```python
from build123d import *

# Parameters (mm, degrees)
SKETCH1_W                = 125
SKETCH1_H                = 125
BOSS_EXTRUDE1_DEPTH      = 2.5
SKETCH3_W                = 125
SKETCH3_H                = 100
BOSS_EXTRUDE3_DEPTH      = 2.5
SKETCH2_W                = 125
SKETCH2_H                = 100
BOSS_EXTRUDE4_DEPTH      = 2.5
SKETCH5_W                = 125
SKETCH5_H                = 102.5
BOSS_EXTRUDE6_DEPTH      = 2.5
SKETCH11_W               = 8
SKETCH11_H               = 1.5
BOSS_EXTRUDE9_DEPTH      = 3
SKETCH12_W               = 8
SKETCH12_H               = 1.5
BOSS_EXTRUDE10_DEPTH     = 4.5
MIRROR10_COPY_1_SKETCH_W = 8
MIRROR10_COPY_1_SKETCH_H = 1.5
MIRROR10_COPY_1_DEPTH    = 3
MIRROR10_COPY_2_SKETCH_W = 8
MIRROR10_COPY_2_SKETCH_H = 1.5
MIRROR10_COPY_2_DEPTH    = 3
MIRROR11_COPY_1_SKETCH_W = 8
MIRROR11_COPY_1_SKETCH_H = 1.5
MIRROR11_COPY_1_DEPTH    = 4.5
MIRROR11_COPY_2_SKETCH_W = 8
MIRROR11_COPY_2_SKETCH_H = 1.5
MIRROR11_COPY_2_DEPTH    = 4.5
SKETCH13_W               = 3
SKETCH13_H               = 75
CUT_EXTRUDE3_DEPTH       = 4.5
SKETCH15_W               = 3
SKETCH15_H               = 75
CUT_EXTRUDE4_DEPTH       = 4.5
SKETCH17_W               = 3
SKETCH17_H               = 75
CUT_EXTRUDE5_DEPTH       = 4.5
SKETCH18_R               = 1.5
CUT_EXTRUDE6_DEPTH       = 4.5
SKETCH19_R               = 1.5
CUT_EXTRUDE7_DEPTH       = 4.5
SKETCH21_R               = 1.5
CUT_EXTRUDE8_DEPTH       = 4.5
SKETCH20_R               = 1.5
CUT_EXTRUDE9_DEPTH       = 4.5
SKETCH22_R               = 1.5
CUT_EXTRUDE10_DEPTH      = 4.5
SKETCH23_R               = 1.5
CUT_EXTRUDE11_DEPTH      = 4.5
SKETCH24_W               = 125
SKETCH24_H               = 125
BOSS_EXTRUDE11_DEPTH     = 2.5
SKETCH25_W               = 10
SKETCH25_H               = 10
BOSS_EXTRUDE12_DEPTH     = 2.5
SKETCH26_W               = 10
SKETCH26_H               = 10
BOSS_EXTRUDE13_DEPTH     = 2.5
SKETCH27_R               = 1.5
CUT_EXTRUDE12_DEPTH      = 2.5
SKETCH28_R               = 1.5
CUT_EXTRUDE13_DEPTH      = 2.5
SKETCH31_R               = 1.75
CUT_EXTRUDE14_DEPTH      = 10
SKETCH29_R               = 1.75
CUT_EXTRUDE15_DEPTH      = 10
SKETCH32_R               = 1.75
CUT_EXTRUDE16_DEPTH      = 10
FILLET1_R                = 5
FILLET2_R                = 5
SKETCH33_R               = 3.75
CUT_EXTRUDE17_DEPTH      = 10


with BuildPart() as part:
    # Sketch1 → Boss-Extrude1 (new body)
    with BuildSketch(Plane(origin=(0, 0, 0), x_dir=(1, 0, 0), z_dir=(0, 1, 0))):
        Rectangle(SKETCH1_W, SKETCH1_H)
    extrude(amount=BOSS_EXTRUDE1_DEPTH)

    # Sketch3 → Boss-Extrude3 (add)
    with BuildSketch(Plane(origin=(0, 0, -62.5), x_dir=(-1, 0, 0), z_dir=(0, 0, -1))):
        with Locations((0, 52.5)):
            Rectangle(SKETCH3_W, SKETCH3_H)
    extrude(amount=-BOSS_EXTRUDE3_DEPTH)

    # Sketch2 → Boss-Extrude4 (add)
    with BuildSketch(Plane.XY.offset(62.5)):
        with Locations((0, 52.5)):
            Rectangle(SKETCH2_W, SKETCH2_H)
    extrude(amount=-BOSS_EXTRUDE4_DEPTH)

    # Sketch5 → Boss-Extrude6 (add)
    with BuildSketch(Plane(origin=(62.5, 0, 0), x_dir=(0, 0, -1), z_dir=(1, 0, 0))):
        with Locations((0, 51.25)):
            Rectangle(SKETCH5_W, SKETCH5_H)
    extrude(amount=-BOSS_EXTRUDE6_DEPTH)

    # Sketch11 → Boss-Extrude9 (add)
    with BuildSketch(Plane(origin=(0, 2.5, 0), x_dir=(1, 0, 0), z_dir=(0, 1, 0))):
        with Locations((54, 50.75)):
            Rectangle(SKETCH11_W, SKETCH11_H)
    boss_extrude9 = extrude(amount=BOSS_EXTRUDE9_DEPTH)

    # Mirror6: Boss-Extrude9 across plane
    add(boss_extrude9.mirror(Plane.XY))

    # Sketch12 → Boss-Extrude10 (add)
    with BuildSketch(Plane.XY.offset(-50)):
        with Locations((54, 4.75)):
            Rectangle(SKETCH12_W, SKETCH12_H)
    boss_extrude10 = extrude(amount=BOSS_EXTRUDE10_DEPTH)

    # Mirror7: Boss-Extrude10 across plane
    add(boss_extrude10.mirror(Plane.XY))

    # Mirror8: Boss-Extrude9 across plane
    add(boss_extrude9.mirror(Plane(origin=(0, 0, 0), x_dir=(0, 0, 1), z_dir=(1, 0, 0))))

    # Mirror9: Boss-Extrude10 across plane
    add(boss_extrude10.mirror(Plane(origin=(0, 0, 0), x_dir=(0, 0, 1), z_dir=(1, 0, 0))))

    # Mirror10 copy 1 sketch → Mirror10 copy 1 (add)
    with BuildSketch(Plane(origin=(0, 2.5, 0), x_dir=(-1, 0, 0), z_dir=(0, 1, 0))):
        with Locations((54, 50.75)):
            Rectangle(MIRROR10_COPY_1_SKETCH_W, MIRROR10_COPY_1_SKETCH_H)
    extrude(amount=MIRROR10_COPY_1_DEPTH)

    # Mirror10 copy 2 sketch → Mirror10 copy 2 (add)
    with BuildSketch(Plane(origin=(0, 2.5, 0), x_dir=(1, 0, 0), z_dir=(0, 1, 0))):
        with Locations((54, -50.75)):
            Rectangle(MIRROR10_COPY_2_SKETCH_W, MIRROR10_COPY_2_SKETCH_H)
    extrude(amount=MIRROR10_COPY_2_DEPTH)

    # Mirror11 copy 1 sketch → Mirror11 copy 1 (add)
    with BuildSketch(Plane(origin=(0, 0, 50), x_dir=(-1, 0, 0), z_dir=(0, 0, -1))):
        with Locations((54, 4.75)):
            Rectangle(MIRROR11_COPY_1_SKETCH_W, MIRROR11_COPY_1_SKETCH_H)
    extrude(amount=MIRROR11_COPY_1_DEPTH)

    # Mirror11 copy 2 sketch → Mirror11 copy 2 (add)
    with BuildSketch(Plane(origin=(0, 0, 50), x_dir=(1, 0, 0), z_dir=(0, 0, -1))):
        with Locations((54, -4.75)):
            Rectangle(MIRROR11_COPY_2_SKETCH_W, MIRROR11_COPY_2_SKETCH_H)
    extrude(amount=MIRROR11_COPY_2_DEPTH)

    # Sketch13 → Cut-Extrude3 (cut)
    with BuildSketch(Plane(origin=(62.5, 0, -52.868964846), x_dir=(0, 0, -1), z_dir=(1, 0, 0))):
        with Locations((-61.5, 52.5)):
            Rectangle(SKETCH13_W, SKETCH13_H)
    cut_extrude3 = extrude(amount=-CUT_EXTRUDE3_DEPTH, mode=Mode.SUBTRACT)

    # Sketch15 → Cut-Extrude4 (cut)
    with BuildSketch(Plane(origin=(62.5, 0, 0), x_dir=(0, 0, -1), z_dir=(1, 0, 0))):
        with Locations((-43.5, 52.5)):
            Rectangle(SKETCH15_W, SKETCH15_H)
    cut_extrude4 = extrude(amount=-CUT_EXTRUDE4_DEPTH, mode=Mode.SUBTRACT)

    # Sketch17 → Cut-Extrude5 (cut)
    with BuildSketch(Plane(origin=(62.5, 0, 0), x_dir=(0, 0, -1), z_dir=(1, 0, 0))):
        with Locations((-26, 52.5)):
            Rectangle(SKETCH17_W, SKETCH17_H)
    cut_extrude5 = extrude(amount=-CUT_EXTRUDE5_DEPTH, mode=Mode.SUBTRACT)

    # Mirror12: Cut-Extrude5 across plane
    add(cut_extrude5.mirror(Plane.XY), mode=Mode.SUBTRACT)

    # Mirror13: Cut-Extrude4 across plane
    add(cut_extrude4.mirror(Plane.XY), mode=Mode.SUBTRACT)

    # Mirror14: Cut-Extrude3 across plane
    add(cut_extrude3.mirror(Plane.XY), mode=Mode.SUBTRACT)

    # Sketch18 → Cut-Extrude6 (cut)
    with BuildSketch(Plane(origin=(62.5, 0, 0), x_dir=(0, 0, -1), z_dir=(1, 0, 0))):
        with Locations((-8.631035154, 90)):
            Circle(SKETCH18_R)
    cut_extrude6 = extrude(amount=-CUT_EXTRUDE6_DEPTH, mode=Mode.SUBTRACT)

    # Sketch19 → Cut-Extrude7 (cut)
    with BuildSketch(Plane(origin=(62.5, 0, 0), x_dir=(0, 0, -1), z_dir=(1, 0, 0))):
        with Locations((-8.631035154, 15)):
            Circle(SKETCH19_R)
    cut_extrude7 = extrude(amount=-CUT_EXTRUDE7_DEPTH, mode=Mode.SUBTRACT)

    # Sketch21 → Cut-Extrude8 (cut)
    with BuildSketch(Plane(origin=(62.5, 0, 0), x_dir=(0, 0, -1), z_dir=(1, 0, 0))):
        with Locations((-26, 15)):
            Circle(SKETCH21_R)
    cut_extrude8 = extrude(amount=-CUT_EXTRUDE8_DEPTH, mode=Mode.SUBTRACT)

    # Sketch20 → Cut-Extrude9 (cut)
    with BuildSketch(Plane(origin=(62.5, 0, 0), x_dir=(0, 0, -1), z_dir=(1, 0, 0))):
        with Locations((-43.5, 15)):
            Circle(SKETCH20_R)
    cut_extrude9 = extrude(amount=-CUT_EXTRUDE9_DEPTH, mode=Mode.SUBTRACT)

    # Mirror15: Cut-Extrude7 across plane
    add(cut_extrude7.mirror(Plane.XY), mode=Mode.SUBTRACT)

    # Mirror16: Cut-Extrude9 across plane
    add(cut_extrude9.mirror(Plane.XY), mode=Mode.SUBTRACT)

    # Mirror17: Cut-Extrude8 across plane
    add(cut_extrude8.mirror(Plane.XY), mode=Mode.SUBTRACT)

    # Sketch22 → Cut-Extrude10 (cut)
    with BuildSketch(Plane(origin=(62.5, 0, 0), x_dir=(0, 0, -1), z_dir=(1, 0, 0))):
        with Locations((-43.5, 90)):
            Circle(SKETCH22_R)
    cut_extrude10 = extrude(amount=-CUT_EXTRUDE10_DEPTH, mode=Mode.SUBTRACT)

    # Sketch23 → Cut-Extrude11 (cut)
    with BuildSketch(Plane(origin=(62.5, 0, 0), x_dir=(0, 0, -1), z_dir=(1, 0, 0))):
        with Locations((-26, 90)):
            Circle(SKETCH23_R)
    cut_extrude11 = extrude(amount=-CUT_EXTRUDE11_DEPTH, mode=Mode.SUBTRACT)

    # Mirror18: Cut-Extrude10 across plane
    add(cut_extrude10.mirror(Plane.XY), mode=Mode.SUBTRACT)

    # Mirror19: Cut-Extrude6 across plane
    add(cut_extrude6.mirror(Plane.XY), mode=Mode.SUBTRACT)

    # Mirror20: Cut-Extrude11 across plane
    add(cut_extrude11.mirror(Plane.XY), mode=Mode.SUBTRACT)

    # Sketch24 → Boss-Extrude11 (add)
    with BuildSketch(Plane(origin=(0, 102.5, 0), x_dir=(1, 0, 0), z_dir=(0, 1, 0))):
        Rectangle(SKETCH24_W, SKETCH24_H)
    extrude(amount=BOSS_EXTRUDE11_DEPTH)

    # Sketch25 → Boss-Extrude12 (add)
    with BuildSketch(Plane.ZY.offset(62.5)):
        with Locations((-57.5, 100)):
            Rectangle(SKETCH25_W, SKETCH25_H)
    boss_extrude12 = extrude(amount=-BOSS_EXTRUDE12_DEPTH)

    # Mirror21: Boss-Extrude12 across plane
    add(boss_extrude12.mirror(Plane.XY))

    # Sketch26 → Boss-Extrude13 (add)
    with BuildSketch(Plane.ZY.offset(62.5)):
        with Locations((-57.5, 5)):
            Rectangle(SKETCH26_W, SKETCH26_H)
    boss_extrude13 = extrude(amount=-BOSS_EXTRUDE13_DEPTH)

    # Mirror22: Boss-Extrude13 across plane
    add(boss_extrude13.mirror(Plane.XY))

    # Sketch27 → Cut-Extrude12 (cut)
    with BuildSketch(Plane.ZY.offset(62.5)):
        with Locations((-56.5, 99)):
            Circle(SKETCH27_R)
    cut_extrude12 = extrude(amount=-CUT_EXTRUDE12_DEPTH, mode=Mode.SUBTRACT)

    # Mirror23: Cut-Extrude12 across plane
    add(cut_extrude12.mirror(Plane.XY), mode=Mode.SUBTRACT)

    # Sketch28 → Cut-Extrude13 (cut)
    with BuildSketch(Plane.ZY.offset(62.5)):
        with Locations((-56.5, 6)):
            Circle(SKETCH28_R)
    cut_extrude13 = extrude(amount=-CUT_EXTRUDE13_DEPTH, mode=Mode.SUBTRACT)

    # Mirror24: Cut-Extrude13 across plane
    add(cut_extrude13.mirror(Plane.XY), mode=Mode.SUBTRACT)

    # Sketch31 → Cut-Extrude14 (cut)
    with BuildSketch(Plane(origin=(62.5, 0, 0), x_dir=(0, 0, -1), z_dir=(1, 0, 0))):
        with Locations((35, 7)):
            Circle(SKETCH31_R)
    extrude(amount=-CUT_EXTRUDE14_DEPTH, mode=Mode.SUBTRACT)

    # Sketch29 → Cut-Extrude15 (cut)
    with BuildSketch(Plane(origin=(62.5, 0, 0), x_dir=(0, 0, -1), z_dir=(1, 0, 0))):
        with Locations((25, 7)):
            Circle(SKETCH29_R)
    extrude(amount=-CUT_EXTRUDE15_DEPTH, mode=Mode.SUBTRACT)

    # Sketch32 → Cut-Extrude16 (cut)
    with BuildSketch(Plane(origin=(62.5, 0, 0), x_dir=(0, 0, -1), z_dir=(1, 0, 0))):
        with Locations((45, 7)):
            Circle(SKETCH32_R)
    extrude(amount=-CUT_EXTRUDE16_DEPTH, mode=Mode.SUBTRACT)

    # Fillet1
    fillet1_edges = [part.edges().sort_by_distance(p)[0] for p in [
        (0, 105, 62.5),
    ]]
    fillet(fillet1_edges, radius=FILLET1_R)

    # Fillet2
    fillet2_edges = [part.edges().sort_by_distance(p)[0] for p in [
        (0, 105, -62.5),
    ]]
    fillet(fillet2_edges, radius=FILLET2_R)

    # Sketch33 → Cut-Extrude17 (cut)
    with BuildSketch(Plane(origin=(62.5, 0, 0), x_dir=(0, 0, -1), z_dir=(1, 0, 0))):
        with Locations((55, 7)):
            Circle(SKETCH33_R)
    extrude(amount=-CUT_EXTRUDE17_DEPTH, mode=Mode.SUBTRACT)


solid = part.part
```
Read the model definition and answer for the solid it produces. Units are mm, in the model's axes. A direction names the side the tool comes from. Give positions to 0.01 mm unless a question says otherwise; leave off trailing zeros. Order: outer loops, then holes, each group sorted by start corner. A loop starts at its lowest first (then second) coordinate and runs counter-clockwise, first axis right, second up. Notation, with made-up numbers: (58.25, 6) -> (63.25, 6) arc R26 cw to (63.25, 38) -> close; hole circle Ø5 at (79, 73). An arc over 180 degrees is marked (long way). One line per item, written item: value. Start each with the question number.
(1) The part is cut by section A-A (x = -46). Determine the outline of the cut face in (y, z), and give its area (3 significant figures).
(2) The part is cut by section B-B (y = 74). State how many separate pieces and enclosed holes the cut face has, and give its area (3 significant figures).
(3) For a pull along Y with two mould halves and no side action, classify faces 1 (the flat face through (-1, 49, 62.5)), 2 (the flat face through (54, 5.5, -49)), 3 (the flat face through (60, 53, 1)), 4 (the cylindrical face through (0.88, 103.5, 61.07)) as released by +Y, released by -Y, zero draft, split by the parting line, or undercut.
(4) Straight lines are drawn through the part: L1, parallel to Z at x = -60.8, y = 99; L2, parallel to Y at x = 62.05, z = -35; L3, parallel to Z at x = -42.5, y = 15.5. For each, find the intervals that lie inside material, in ascending order.
(5) A flat-ended cylindrical pin translates along its axis: P1, Ø1, axis at y = 24, z = 37.5, coming from the -X side. Find the tip coordinate at first contact, or state that the pin passes through.
(6) A tool of negligible diameter and unlimited length cuts with its end or side. For faces 5 (the flat face through (-60, 98.8, -54.6)), 6 (the flat face through (-54, 4, -48)), 7 (the flat face through (-1, 0, -1)), from which of +Z, -Z, +X, -X, +Y, -Y can it reach the whole face along a straight path? Write none if from no direction.
(7) The part is cut by section C-C (z = 14.5). Determine the outline of the cut face in (x, y).
Taken from the geometry:
1. outline: (0, -62.5) -> (100, -62.5) arc R5 ccw to (105, -57.5) -> (105, 57.5) arc R5 ccw to (100, 62.5) -> (0, 62.5) -> close; hole (2.5, -60) -> (102.5, -60) -> (102.5, 60) -> (2.5, 60) -> close
1. area: 1,110 mm^2
2. separate pieces: 7
2. enclosed holes: 0
2. area: 880 mm^2
3. face 1: zero draft
3. face 2: undercut
3. face 3: undercut
3. face 4: released by +Y
4. L1: -62.5 to -58, -55 to -52.5, 52.5 to 55, 58 to 62.5
4. L2: 0 to 5.25, 8.75 to 105
4. L3: -62.5 to -60, 60 to 62.5
5. P1: x = 60
6. face 5: none
6. face 6: -X
6. face 7: +Z, -Z, +X, -X, -Y
7. outline: (-62.5, 0) -> (62.5, 0) -> (62.5, 105) -> (-62.5, 105) -> (-62.5, 102.5) -> (60, 102.5) -> (60, 2.5) -> (-62.5, 2.5) -> close
